The listing builds one solid part. Answer for the finished solid, in the listing's coordinates (mm). A direction names the side the tool comes from. Give positions to 0.01 mm unless a question says otherwise; leave off trailing zeros. Loops run counter-clockwise (first coordinate to the right, second up) from the corner with the lowest first, then second, coordinate; pieces in that order, holes last.
Item 1: A tool of negligible diameter and unlimited length cuts with its end or side. For faces 5 (the face through (-1, 0, 18)), 6 (the face through (10, 0, 20)), from which of +Z, -Z, +X, -X, +Y, -Y can it reach the whole face along a straight path? Write none if from no direction.
Item 2: Each of these flat-tipped pins is pushed along its axis until it touches: pin 1 Ø10 at (y, z) = (-11.5, 7) entering from -X; pin 2 Ø5.5 at (y, z) = (0, 18) entering from -X; pin 3 Ø12 at (x, z) = (-4, 7) entering from +Y. Where does it stop, or does it pass through?
Item 3: Section A-A, the plane y = 3.5 is taken. Give the vertices of the cut face in (x, z).
Item 4: Section C-C, the plane x = 0 is taken. Give the vertices of the cut face in (y, z).
Item 5: Consider line 1 along X through (y, z) = (20, 15.25); line 2 along X through (y, z) = (15, 19.25); line 3 along Y through (x, z) = (-15.5, 8.5). Determine where each line is inside the solid, lowest interval first.
Item 6: Section B-B, the plane z = 9.5 is taken. Give the vertices of the cut face in (x, y), and give its area (3 significant figures).
Item 7: The mould has two halves that part along X. Classify faces 1 (the face through (0, 0, 15)), 2 (the face through (1, 0, 18)), 3 (the face through (23.846, 7.509, 9.86)), 4 (the face through (0, 0, 0)): pulls with the +X half, pulls with the -X half, needs draft (parallel to the pull), parting line crosses it, or undercut.
Item 8: Section D-D, the plane x = -5 is taken. Give the vertices of the cut face in (y, z), and give its area (3 significant figures).
from build123d import *

# Parameters (mm, degrees)
SKETCH1_R           = 25
BOSS_EXTRUDE1_DEPTH = 20
SKETCH2_W           = 2
SKETCH2_H           = 50
CUT_EXTRUDE1_DEPTH  = 5


with BuildPart() as part:
    # Sketch1 → Boss-Extrude1 (new body)
    with BuildSketch(Plane.XY):
        Circle(SKETCH1_R)
    extrude(amount=BOSS_EXTRUDE1_DEPTH)

    # Sketch2 → Cut-Extrude1 (cut)
    with BuildSketch(Plane.XY.offset(20)):
        Rectangle(SKETCH2_W, SKETCH2_H)
    extrude(amount=-CUT_EXTRUDE1_DEPTH, mode=Mode.SUBTRACT)


solid = part.part
Worked answers:
1. face 5: +Z, +Y, -Y
1. face 6: +Z, +X, -X, +Y, -Y
2. pin 1: stops at x = -24.14
2. pin 2: stops at x = -25
2. pin 3: stops at y = 25
3. outline: (-24.75, 0) - (24.75, 0) - (24.75, 20) - (1, 20) - (1, 15) - (-1, 15) - (-1, 20) - (-24.75, 20) - close
4. outline: (-25, 0) - (25, 0) - (25, 15) - (-25, 15) - close
5. line 1: x = -15 to -1, 1 to 15
5. line 2: x = -20 to -1, 1 to 20
5. line 3: y = -19.62 to 19.62
6. outline: circle Ø50 at (0, 0)
6. area: 1,960 mm2
7. face 1: undercut
7. face 2: undercut
7. face 3: parting line crosses it
7. face 4: needs draft
8. outline: (-24.49, 0) - (24.49, 0) - (24.49, 20) - (-24.49, 20) - close
8. area: 980 mm2
